The listing builds one solid part. Answer for the finished solid, in the listing's coordinates (mm). A direction names the side the tool comes from. Coordinates: 2 decimals unless noted, no trailing zeros. Loops run counter-clockwise (first coordinate to the right, second up) from the corner with the lowest first, then second, coordinate; pieces in that order, holes last. Notation, with made-up numbers: (29, -2.5) - (65, -2.5) arc R13 cw to (65, 6.5) - close; hole circle Ø10 at (81, 89.25). An arc over 180 degrees is marked (long way). Put each result on its own line as item: value.
```python
from build123d import *

# Parameters (mm, degrees)
SKETCH3_W                = 25.4
SKETCH3_H                = 25.4
SKETCH3_W_2              = 22.225
SKETCH3_H_2              = 22.225
BOSS_EXTRUDE1_DEPTH      = 76.2
BOSS_EXTRUDE1_DEPTH_BACK = 76.2
SKETCH4_W                = 25.4
SKETCH4_H                = 25.4
SKETCH4_W_2              = 22.225
SKETCH4_H_2              = 22.225
CUT_EXTRUDE1_DEPTH       = 3.175


with BuildPart() as part:
    # Sketch3 → Boss-Extrude1 (new body, two sides)
    with BuildSketch(Plane.XY) as boss_extrude1_sk:
        Rectangle(SKETCH3_W, SKETCH3_H)
        Rectangle(SKETCH3_W_2, SKETCH3_H_2, mode=Mode.SUBTRACT)
    extrude(amount=BOSS_EXTRUDE1_DEPTH)
    extrude(boss_extrude1_sk.sketch, amount=-BOSS_EXTRUDE1_DEPTH_BACK)

    # Sketch4 → Cut-Extrude1 (cut)
    with BuildSketch(Plane(origin=(0, 0, -76.2), x_dir=(-1, 0, 0), z_dir=(0, 0, -1))):
        Rectangle(SKETCH4_W, SKETCH4_H)
        Rectangle(SKETCH4_W_2, SKETCH4_H_2, mode=Mode.SUBTRACT)
    extrude(amount=-CUT_EXTRUDE1_DEPTH, mode=Mode.SUBTRACT)


solid = part.part
```
1) This flat-tipped pin is pushed along its axis until it touches: pin 1 (1.5 mm diameter, centred on x = -8.5, y = 3, fed in from +Z). Where does it stop, or does it pass through?
Found:
pin 1: passes through
2) For faces 5 (the face through (-11.112, 0, 3)), 6 (the face through (-12.7, 0, 3)), determine the directions among +Z, -Z, +X, -X, +Y, -Y from which every point of the face is accessible in a straight line to the end or side of a thin tool.
Found:
face 5: +Z, -Z
face 6: +Z, -Z, -X, +Y, -Y
3) The part is cut by section A-A (x = -3.5). Give the vertices of the cut face in (y, z) (1 decimal).
Found:
outline: (-12.7, -73) - (-11.1, -73) - (-11.1, 76.2) - (-12.7, 76.2) - close; (11.1, -73) - (12.7, -73) - (12.7, 76.2) - (11.1, 76.2) - close
4) The part is cut by section C-C (z = -52.5). Give the vertices of the cut face in (x, y).
Found:
outline: (-12.7, -12.7) - (12.7, -12.7) - (12.7, 12.7) - (-12.7, 12.7) - close; hole (-11.11, -11.11) - (11.11, -11.11) - (11.11, 11.11) - (-11.11, 11.11) - close
5) A straight line is drawn through the part: L1, parallel to Y at x = 9.5, z = 48. Find the intervals that lie inside material, in ascending order. Write a range as [from, to].
Found:
L1: y = [-12.7, -11.11], [11.11, 12.7]
6) For a pull along Y with two mould halves and no side action, classify faces 1 (the face through (0, -11.112, 3)), 2 (the face through (0, -12.7, 3)), 3 (the face through (-11.3, 0.1, 76.2)), 4 (the face through (0, 12.7, 3)) as pulls with the +Y half, pulls with the -Y half, needs draft (parallel to the pull), parting line crosses it, or undercut.
Found:
face 1: undercut
face 2: pulls with the -Y half
face 3: needs draft
face 4: pulls with the +Y half
